Verification items for the finished model (mm, model axes). A direction names the side the tool comes from. Round coordinates to 2 decimals unless told otherwise and drop trailing zeros. Write each loop counter-clockwise with the first axis right and the second up, starting at its lowest first coordinate (ties: lowest second). Pieces come first, ordered by that corner, then holes. Notation, with made-up numbers: M 37.5,-25.75 L 61.5,-25.75 A30 ccw 61.5,7.25 Z; hole C -31,46 d4. An arc over 180 degrees is marked long. One line per item, written item: value. Start each with the question number.
Item 1: Gauge pin test, flat ends, axial feed: pin 1 (4.5 mm diameter, centred on x = -18, y = -16, fed in from -Z); pin 2 (6 mm diameter, centred on x = -7, y = 6.5, fed in from +Z); pin 3 (5 mm diameter, centred on y = 17.5, z = 10.5, fed in from -X); pin 4 (8 mm diameter, centred on x = 10.5, y = 7, fed in from +Z). Record the tip position at first contact, or that the pin passes through.
Item 2: Section check A-A, the plane x = -10. Record the cut outline in (y, z), then the cut area to 3 significant figures.
Item 3: Tool access check on faces 4 (the face through (-10, 0, 15)), 5 (the face through (5, 12.8, 24)), 6 (the face through (-18, -13.7, 11.8)). Record the directions out of +Z, -Z, +X, -X, +Y, -Y that give a thin tool (end or side, any length) a straight path to the whole face; none if there is none.
Item 4: Section check B-B, the plane z = 2.5. Record the cut outline in (x, y), then the cut area to 3 significant figures.
Item 5: Thickness scan on probe 1 along Y at (x, z) = (-15, 9.5); probe 2 along Z at (x, y) = (2.5, -15); probe 3 along Z at (x, y) = (-12.5, 10). Record the ranges inside material, lowest first. Write a range as from..to.
Item 6: Draft check along Y on faces 1 (the face through (8.7, -0.3, 27.6)), 2 (the face through (5, -17.2, 24)), 3 (the face through (0, -22.5, 9)). Enter one of: +Y half, -Y half, draft (parallel to the pull), parting line (faces both ways), or undercut.
Item 7: Section check D-D, the plane y = -4.5. Record the cut outline in (x, z), then the cut area to 3 significant figures.
Item 8: Section check C-C, the plane x = 7. Record the cut outline in (y, z), then the cut area to 3 significant figures.
from build123d import *

# Parameters (mm, degrees)
SKETCH_W        = 40
SKETCH_H        = 45
PAD_DEPTH       = 35
POCKET_DEPTH    = 45.001
SKETCH002_R     = 2.25
POCKET001_DEPTH = 15.001
SKETCH003_R     = 2.25
POCKET002_DEPTH = 20.001
SKETCH004_R     = 4.75
POCKET003_DEPTH = 15
POCKET004_DEPTH = 4
SKETCH006_R     = 2.25
POCKET005_DEPTH = 7


with BuildPart() as part:
    # Sketch → Pad (new body)
    with BuildSketch(Plane.XY):
        Rectangle(SKETCH_W, SKETCH_H)
    extrude(amount=PAD_DEPTH)

    # Sketch001 → Pocket (cut, through all)
    with BuildSketch(Plane.XZ.offset(22.5)):
        Polygon((-21, 15), (0, 15), (0, 35), (5, 35), (12.5, 20), (21, 20), (21, 36), (-21, 36), align=None)
    extrude(amount=-POCKET_DEPTH, mode=Mode.SUBTRACT)

    # Sketch002 → Pocket001 (cut, through all)
    with BuildSketch(Plane.XY.offset(15)):
        with Locations((-10, 15)):
            Circle(SKETCH002_R)
        with Locations((-10, -15)):
            Circle(SKETCH002_R)
    extrude(amount=-POCKET001_DEPTH, mode=Mode.SUBTRACT)

    # Sketch003 → Pocket002 (cut, through all)
    with BuildSketch(Plane(origin=(0, 0, 0), x_dir=(0, -1, 0), z_dir=(-1, 0, 0))):
        with Locations((-15, 25)):
            Circle(SKETCH003_R)
        with Locations((15, 25)):
            Circle(SKETCH003_R)
    extrude(amount=-POCKET002_DEPTH, mode=Mode.SUBTRACT)

    # Sketch004 → Pocket003 (cut)
    with BuildSketch(Plane.YZ.offset(20)):
        with Locations((-15, 25)):
            Circle(SKETCH004_R)
        with Locations((15, 25)):
            Circle(SKETCH004_R)
    extrude(amount=-POCKET003_DEPTH, mode=Mode.SUBTRACT)

    # Sketch005 → Pocket004 (cut)
    with BuildSketch(Plane(origin=(-20, 0, 0), x_dir=(0, -1, 0), z_dir=(-1, 0, 0))):
        Polygon((-18.720726, 13.5), (-14.679274, 13.5), (-12.658548, 10), (-14.679274, 6.5), (-18.720726, 6.5), (-20.741452, 10), align=None)
        Polygon((12.658548, 10), (14.679274, 6.5), (18.720726, 6.5), (20.741452, 10), (18.720726, 13.5), (14.679274, 13.5), align=None)
    extrude(amount=-POCKET004_DEPTH, mode=Mode.SUBTRACT)

    # Sketch006 → Pocket005 (cut)
    with BuildSketch(Plane(origin=(-20, 0, 0), x_dir=(0, -1, 0), z_dir=(-1, 0, 0))):
        with Locations((-16.7, 10)):
            Circle(SKETCH006_R)
        with Locations((16.7, 10)):
            Circle(SKETCH006_R)
    extrude(amount=-POCKET005_DEPTH, mode=Mode.SUBTRACT)


solid = part.part
Response values:
1. pin 1: stops at z = 0
1. pin 2: stops at z = 15
1. pin 3: stops at x = -16
1. pin 4: stops at z = 32
2. outline: M -22.5,0 L -17.25,0 L -17.25,15 L -22.5,15 Z; M -12.75,0 L 12.75,0 L 12.75,15 L -12.75,15 Z; M 17.25,0 L 22.5,0 L 22.5,15 L 17.25,15 Z
2. area: 540 mm2
3. face 4: +Z, -X, +Y, -Y
3. face 5: +X
3. face 6: -X
4. outline: M -20,-22.5 L 20,-22.5 L 20,22.5 L -20,22.5 Z; hole C -10,-15 d4.5; hole C -10,15 d4.5
4. area: 1,770 mm2
5. probe 1: y = -22.5..-18.89, -14.51..14.51, 18.89..22.5
5. probe 2: z = 0..22.75, 27.25..35
5. probe 3: z = 0..15
6. face 1: draft
6. face 2: undercut
6. face 3: -Y half
7. outline: M -20,0 L 20,0 L 20,20 L 12.5,20 L 5,35 L 0,35 L 0,15 L -20,15 Z
7. area: 831 mm2
8. outline: M -22.5,0 L 22.5,0 L 22.5,31 L -22.5,31 Z; hole C -15,25 d9.5; hole C 15,25 d9.5
8. area: 1,250 mm2
